Source: CAD feature listing. Evaluate the final solid. Frame: model axes, mm. Face numbers are marked on the shaded views. A direction names the side the tool comes from. Coordinates: 2 decimals unless noted, no trailing zeros. Write each loop counter-clockwise with the first axis right and the second up, starting at its lowest first coordinate (ties: lowest second). Pieces come first, ordered by that corner, then holes. Notation, with made-up numbers: (43, 6) -> (54, 6) arc R9 cw to (54, 19) -> close; hole circle Ø7 at (24.25, 20). An arc over 180 degrees is marked (long way). One line per item, written item: value. Start each with the question number.
1. Section query C-C, the plane x = -7. Output: boundary loops of the cut face in (y, z).
2. Section query D-D, the plane y = -11.75. Output: boundary loops of the cut face in (x, z).
3. Section query A-A, the plane x = -19. Output: boundary loops of the cut face in (y, z), and give its area (3 significant figures).
4. Section query B-B, the plane z = -2. Output: boundary loops of the cut face in (x, y).
5. Access query for the marked faces 1, 2, 3, 4 and 5. Directions: +Z, -Z, +X, -X, +Y, -Y. A direction counts if a zero-diameter tool reaches every point of the face in a straight line with its end or side. Return the directions, or none.
6. Line query: line 1 (Z direction, x = 8, y = 4.75); line 2 (Z direction, x = -0.5, y = 3.75); line 3 (Y direction, x = 4, z = -21). Output: solid intervals per line, ascending.
7. First-contact query: P1, Ø10, axis at x = -14, z = 16, coming from the -Y side; P2, Ø3, axis at x = 17, y = -10.5, coming from the -Z side; P3, Ø5, axis at x = 19, y = -6.5, coming from the +Z side. Flat tips, straight axial feed; report the tip coordinate or a pass-through.
8. Mould query, pull axis Y, two halves, no side actions, for the marked faces 6, 7 and 8. Classes: released by +Y, released by -Y, zero draft, split by the parting line, or undercut.
from build123d import *

# Parameters (mm, degrees)
SKETCH3_W           = 44
SKETCH3_H           = 47
BOSS_EXTRUDE1_DEPTH = 6
SKETCH4_W           = 42
SKETCH4_H           = 44
CUT_EXTRUDE1_DEPTH  = 4
SKETCH5_W           = 44
SKETCH5_H           = 3
BOSS_EXTRUDE2_DEPTH = 1.5
SKETCH6_W           = 24
SKETCH6_H           = 12
CUT_EXTRUDE2_DEPTH  = 2
BOSS_EXTRUDE3_START = 22
BOSS_EXTRUDE3_DEPTH = 10
FILLET1_R           = 3
FILLET2_R           = 1


with BuildPart() as part:
    # Sketch3 → Boss-Extrude1 (new body)
    with BuildSketch(Plane(origin=(0, 0, 0), x_dir=(1, 0, 0), z_dir=(0, 1, 0))):
        Rectangle(SKETCH3_W, SKETCH3_H)
    extrude(amount=BOSS_EXTRUDE1_DEPTH)

    # Sketch4 → Cut-Extrude1 (cut)
    with BuildSketch(Plane(origin=(0, 6, 0), x_dir=(1, 0, 0), z_dir=(0, 1, 0))):
        with Locations((-1, 0)):
            Rectangle(SKETCH4_W, SKETCH4_H)
    extrude(amount=-CUT_EXTRUDE1_DEPTH, mode=Mode.SUBTRACT)

    # Sketch5 → Boss-Extrude2 (add)
    with BuildSketch(Plane(origin=(0, 6, 0), x_dir=(1, 0, 0), z_dir=(0, 1, 0))):
        with Locations((0, 22)):
            Rectangle(SKETCH5_W, SKETCH5_H)
    boss_extrude2 = extrude(amount=-BOSS_EXTRUDE2_DEPTH)

    # Mirror1: Boss-Extrude2 across plane
    add(boss_extrude2.mirror(Plane.XY))

    # Sketch6 → Cut-Extrude2 (cut)
    with BuildSketch(Plane.XZ):
        with Locations((-22, -11.5)):
            Rectangle(SKETCH6_W, SKETCH6_H)
    extrude(amount=-CUT_EXTRUDE2_DEPTH, mode=Mode.SUBTRACT)

    # Sketch7 → Boss-Extrude3 (add)
    with BuildSketch(Plane(origin=(0, 0, 0), x_dir=(0, 0, -1), z_dir=(1, 0, 0)).offset(BOSS_EXTRUDE3_START)):
        with BuildLine():
            Line((-6.75, -2), (6.75, -2))
            ThreePointArc((6.75, -2), (9.829603655, -7.636154321), (8.962619003, -14))
            Line((8.962619003, -14), (11.5, -14))
            Line((11.5, -14), (11.5, 0))
            Line((11.5, 0), (-11.5, 0))
            Line((-11.5, 0), (-11.5, -14))
            Line((-11.5, -14), (-8.962619003, -14))
            ThreePointArc((-8.962619003, -14), (-9.829603655, -7.636154321), (-6.75, -2))
        make_face()
    extrude(amount=-BOSS_EXTRUDE3_DEPTH)

    # Fillet1
    fillet1_edges = [part.edges().sort_by_distance(p)[0] for p in [
        (17, 0, 11.5),
        (17, 0, -11.5),
    ]]
    fillet(fillet1_edges, radius=FILLET1_R)

    # Fillet2
    fillet2_edges = [part.edges().sort_by_distance(p)[0] for p in [
        (17, -2, 6.75),
        (17, -14, 11.5),
        (17, -14, -11.5),
        (17, -2, -6.75),
    ]]
    fillet(fillet2_edges, radius=FILLET2_R)


solid = part.part
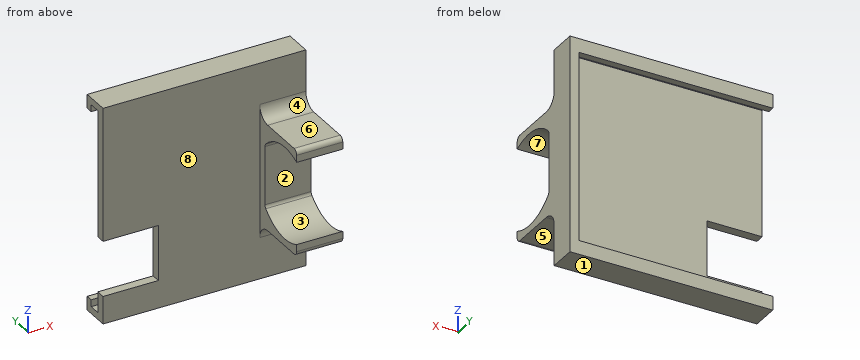
Computed values:
1. outline: (0, -23.5) -> (6, -23.5) -> (6, -20.5) -> (4.5, -20.5) -> (4.5, -22) -> (2, -22) -> (2, 22) -> (4.5, 22) -> (4.5, 20.5) -> (6, 20.5) -> (6, 23.5) -> (0, 23.5) -> close
2. outline: (12, -11.5) -> (22, -11.5) -> (22, -9.75) -> (12, -9.75) -> close; (12, 9.75) -> (22, 9.75) -> (22, 11.5) -> (12, 11.5) -> close
3. outline: (0, -23.5) -> (6, -23.5) -> (6, -20.5) -> (4.5, -20.5) -> (4.5, -22) -> (2, -22) -> (2, -17.5) -> (0, -17.5) -> close; (0, -5.5) -> (2, -5.5) -> (2, 22) -> (4.5, 22) -> (4.5, 20.5) -> (6, 20.5) -> (6, 23.5) -> (0, 23.5) -> close
3. area: 86.5 mm²
4. outline: (-22, 0) -> (12, 0) -> (12, -2) -> (22, -2) -> (22, 6) -> (20, 6) -> (20, 2) -> (-22, 2) -> close
5. face 1: -Z, +X, -X, +Y, -Y
5. face 2: +X, -X, -Y
5. face 3: +X, -X
5. face 4: +Z, +X, -X, -Y
5. face 5: -Z, +X, -X, -Y
6. line 1: z = -23.5 to -20.5, 20.5 to 23.5
6. line 2: z = -23.5 to -22, 22 to 23.5
6. line 3: y = 0 to 2, 4.5 to 6
7. P1: stops at y = 0
7. P2: stops at z = -11.5
7. P3: stops at z = 11.5
8. face 6: zero draft
8. face 7: undercut
8. face 8: released by -Y
